Autodesk Inventor part; units mm, degrees
ref_plane "YZ Plane" through (0, 0, 0) normal (1, 0, 0) x (0, 1, 0)
ref_plane "XZ Plane" through (0, 0, 0) normal (0, 1, 0) x (-1, 0, 0)
ref_plane "XY Plane" through (0, 0, 0) normal (0, 0, 1) x (1, 0, 0)
sketch "Sketch1" plane through (0, 0, 0) normal (0, 1, 0) x (-1, 0, 0)
  line L0 (-1.27, 1.27) -> (1.27, 1.27)
  line L1 (1.27, 1.27) -> (1.27, -1.27)
  line L2 (1.27, -1.27) -> (-1.27, -1.27)
  line L3 (-1.27, -1.27) -> (-1.27, 1.27)
  line L4 (-1.27, 1.27) -> (1.27, -1.27) construction
  line L5 (1.27, 1.27) -> (-1.27, -1.27) construction
  point P0 (0, 0)
  dimension "d0" = 2.54
extrude "Extrusion1" add sketch "Sketch1" along normal blind 2.6035
chamfer "Chamfer1" distance 0.381 angle 45 4 edges at (1.27, 1.3017, 1.27) (-1.27, 1.3017, 1.27) (1.27, 1.3017, -1.27) (-1.27, 1.3017, -1.27)
sketch "Sketch2" plane through (0, 2.6035, 0) normal (0, 1, 0) x (1, 0, 0)
  line L0 (0.2984, 0.2984) -> (-0.2984, 0.2984)
  line L1 (-0.2984, 0.2984) -> (-0.2984, -0.2984)
  line L2 (-0.2984, -0.2984) -> (0.2984, -0.2984)
  line L3 (0.2984, -0.2984) -> (0.2984, 0.2984)
  line L4 (0.2984, 0.2984) -> (-0.2984, -0.2984) construction
  line L5 (-0.2984, 0.2984) -> (0.2984, -0.2984) construction
  point P0 (0, 0)
  dimension "d6" = 0.5969
extrude "Extrusion2" add sketch "Sketch2" along normal blind 6.35 and the other way blind 14.605
chamfer "Chamfer2" distance 0.1905 angle 45 8 edges at (0.2984, 8.9535, 0) (0, 8.9535, -0.2984) (-0.2984, 8.9535, 0) (0, 8.9535, 0.2984) (0, -12.0015, -0.2984) (0.2984, -12.0015, 0) (0, -12.0015, 0.2984) (-0.2984, -12.0015, 0)
sketch "Sketch3" plane through (0, 8.9535, 0) normal (0, 1, 0) x (1, 0, 0)
  circle A0 centre (0, 0) radius 0.0635
  dimension "d14" = 0.127
extrude "Extrusion3" cut sketch "Sketch3" against normal through all
properties part number "Single Long Male Header"
Geometry check sheet. Reference: the model listing, model coordinates, mm. Coordinates: 2 decimals unless noted, no trailing zeros. Order: outer loops, then holes, each group sorted by start corner. A loop starts at its lowest first (then second) coordinate and runs counter-clockwise, first axis right, second up. Notation, with made-up numbers: (47.25, 13.25) - (85.25, 13.25) arc R32 ccw to (85.25, 40.25) - close; hole circle Ø7 at (45.5, -28.5). An arc over 180 degrees is marked (long way). Use one line per item in the form item = value.
1. Section check C-C (x = -0.55). Record the boundary of the cut face in (y, z).
Here are the results:
outline = (0, -1.27) - (2.6, -1.27) - (2.6, 1.27) - (0, 1.27) - close
2. Section check B-B (z = 0.55). Record the boundary of the cut face in (x, y).
Here are the results:
outline = (-1.27, 0) - (1.27, 0) - (1.27, 2.6) - (-1.27, 2.6) - close
3. Scan lines: line 1 (Y direction, x = -0.55, z = 1.15); line 2 (Z direction, x = -0.15, y = -6). Record each from-to range of solid material in increasing order.
Here are the results:
line_1 = 0 to 2.6
line_2 = -0.3 to 0.3
4. Gauge pin test, flat ends, axial feed: pin 1 (1 mm diameter, centred on x = 0, y = -8, fed in from -Z); pin 2 (0.8 mm diameter, centred on x = 0.5, z = 0.5, fed in from +Y); pin 3 (0.5 mm diameter, centred on y = 5, z = 0, fed in from -X). Record the tip position at first contact, or that the pin passes through.
Here are the results:
pin_1 = -0.3
pin_2 = 8.84
pin_3 = -0.3
5. Section check A-A (y = 5.5). Record the boundary of the cut face in (x, z), then the cut area to 3 significant figures.
Here are the results:
outline = (-0.3, -0.3) - (0.3, -0.3) - (0.3, 0.3) - (-0.3, 0.3) - close; hole circle Ø0.13 at (0, 0)
area = 0.344 mm²
